Read the model definition and answer for the solid it produces. Units are mm, in the model's axes. Face numbers are marked on the shaded views. A direction names the side the tool comes from. Coordinates: 2 decimals unless noted, no trailing zeros. Order: outer loops, then holes, each group sorted by start corner. A loop starts at its lowest first (then second) coordinate and runs counter-clockwise, first axis right, second up. Notation, with made-up numbers: M 50,4 L 59,4 A19 ccw 59,12 Z; hole C 85,-6.75 d3. An arc over 180 degrees is marked long. Use a Markdown table: item, result. Add a question column.
1) The mould has two halves that part along Z. Classify the marked faces 1, 2 and 3: released by +Z, released by -Z, zero draft, split by the parting line, or undercut.
2) Find the intervals of material crossed by probe 1 along Z at (x, y) = (-53, 19.5); probe 2 along Y at (x, z) = (-15.5, -103.45); probe 3 along X at (y, z) = (31, -102), in increasing order. Write a range as [from, to].
3) Each of these flat-tipped pins is pushed along its axis until it touches: pin 1 Ø2 at (y, z) = (24.5, 22.5) entering from +X; pin 2 Ø10 at (y, z) = (34.5, -17.5) entering from -X; pin 3 Ø1 at (x, z) = (-12, -74.5) entering from +Y. Where does it stop, or does it pass through?
4) For the marked faces 4 and 5, determine the directions among +Z, -Z, +X, -X, +Y, -Y from which every point of the face is accessible in a straight line to the end or side of a thin tool.
5) Find section B-B on y = 39.5. Write down the section's boundary in (x, z).
6) Find section A-A on x = -53. Write down the section's boundary in (y, z), plus the area to 3 significant figures.
7) Find section C-C on z = -27.5. Write down the section's boundary in (x, y), plus the area to 3 significant figures.
Autodesk Inventor part; units mm, degrees
ref_plane "YZ Plane" through (0, 0, 0) normal (1, 0, 0) x (0, 1, 0)
ref_plane "XZ Plane" through (0, 0, 0) normal (0, 1, 0) x (-1, 0, 0)
ref_plane "XY Plane" through (0, 0, 0) normal (0, 0, 1) x (1, 0, 0)
sketch "Boceto1" plane through (0, 0, 0) normal (0, 1, 0) x (-1, 0, 0)
  line L0 (120, 0) -> (60, -103.923)
  line L1 (60, -103.923) -> (-60, -103.923)
  line L2 (-60, -103.923) -> (-120, 0)
  line L3 (-120, 0) -> (-60, 103.923)
  line L4 (-60, 103.923) -> (60, 103.923)
  line L5 (60, 103.923) -> (120, 0)
  point P0 (0, 0)
  point P1 (0, 0)
  dimension "d0" = 120
extrude "Extrusión1" add sketch "Boceto1" along normal blind 3
sketch "Boceto2" plane through (0, 3, 0) normal (0, 1, 0) x (1, 0, 0)
  line L0 (-60, -103.923) -> (60, -103.923)
  line L1 (60, -103.923) -> (120, 0)
  line L2 (120, 0) -> (60, 103.923)
  line L3 (60, 103.923) -> (-60, 103.923)
  line L4 (-60, 103.923) -> (-120, 0)
  line L5 (-120, 0) -> (-60, -103.923)
  line L6 (-58.8453, -101.923) -> (58.8453, -101.923)
  line L7 (58.8453, -101.923) -> (117.6906, 0)
  line L8 (117.6906, 0) -> (58.8453, 101.923)
  line L9 (58.8453, 101.923) -> (-58.8453, 101.923)
  line L10 (-58.8453, 101.923) -> (-117.6906, 0)
  line L11 (-117.6906, 0) -> (-58.8453, -101.923)
  point P0 (0, 0)
  dimension "d3" = 2
extrude "Extrusión2" add sketch "Boceto2" along normal blind 60
sketch "Boceto5" plane through (120, 0, 0) normal (0.866, 0, 0.5) x (0.5, 0, -0.866)
  line L0 (-120, 0) -> (0, 0)
  line L1 (0, 0) -> (0, 63)
  line L2 (-120, 63) -> (0, 63)
  line L3 (-120, 0) -> (-120, 63)
  point P0 (-60, 0)
sketch "Boceto9" plane through (-60, 0, 103.923) normal (-0.866, 0, 0.5) x (0.5, 0, 0.866)
  circle A0 centre (-117, 58.5) radius 1.5
  circle A1 centre (-3, 58.5) radius 1.5
  point P0 (-60, 0)
extrude "Extrusión7" cut sketch "Boceto9" against normal blind 220
sketch "Boceto10" plane through (-120, 0, 0) normal (-0.866, 0, -0.5) x (-0.5, 0, 0.866)
  line L0 (-120, 0) -> (0, 0)
  line L1 (0, 0) -> (0, 63)
  line L2 (-120, 63) -> (0, 63)
  line L3 (-120, 0) -> (-120, 63)
  line L4 (-120, 63) -> (-120, 31.5)
  line L5 (-120, 31.5) -> (-60, 31.5)
  line L6 (-60, 31.5) -> (-60, 0)
  dimension "d19" = 31.5
  dimension "d20" = 60
sketch "Boceto12" plane through (60, 0, -103.923) normal (0, 0, -1) x (-1, 0, 0)
  line L0 (120, 0) -> (120, 63)
  line L1 (120, 31.5) -> (60, 31.5)
  line L2 (60, 31.5) -> (60, 0)
  dimension "d23" = 60
sketch "Boceto13" plane through (60, 0, -103.923) normal (0, 0, -1) x (-1, 0, 0)
  circle A0 centre (44.5, 31.5) radius 1.25
  circle A1 centre (75.5, 31.5) radius 1.25
  point P0 (60, 0)
extrude "Extrusión9" cut sketch "Boceto13" against normal blind 220
sketch "Boceto14" plane through (60, 0, -103.923) normal (0.866, 0, -0.5) x (-0.5, 0, -0.866)
  line L0 (-60, 0) -> (-60, 31.5)
  line L1 (-60, 31.5) -> (0, 31.5)
  dimension "d26" = 31.5
sketch "Boceto15" plane through (60, 0, -103.923) normal (0.866, 0, -0.5) x (-0.5, 0, -0.866)
  circle A0 centre (-75.5, 31.5) radius 1.25
  circle A1 centre (-44.5, 31.5) radius 1.25
  point P0 (-60, 0)
extrude "Extrusión10" cut sketch "Boceto15" against normal blind 220
sketch "Boceto16" plane through (120, 0, 0) normal (0.866, 0, 0.5) x (0.5, 0, -0.866)
  line L0 (-60, 0) -> (-60, 31.5)
  line L1 (-60, 31.5) -> (0, 31.5)
  line L2 (0, 0) -> (0, 63)
  dimension "d29" = 31.5
sketch "Boceto17" plane through (120, 0, 0) normal (0.866, 0, 0.5) x (0.5, 0, -0.866)
  circle A0 centre (-75.5, 31.5) radius 1.25
  circle A1 centre (-44.5, 31.5) radius 1.25
  point P0 (-60, 0)
extrude "Extrusión11" cut sketch "Boceto17" against normal blind 220
properties part number "BaseHEX"
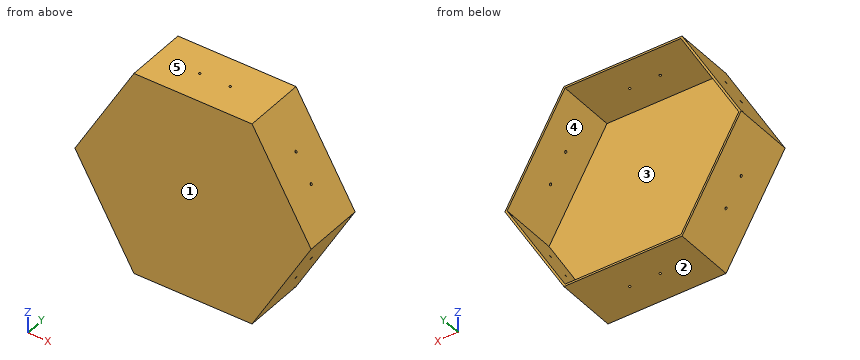
Check result:
| question | item | result |
|---|---|---|
| 1 | face 1 | zero draft |
| 1 | face 2 | released by -Z |
| 1 | face 3 | undercut |
| 2 | probe 1 | z = [-103.92, -101.92], [101.92, 103.92] |
| 2 | probe 2 | y = [0, 30.25], [32.75, 63] |
| 2 | probe 3 | x = [-61.11, -16.65], [-14.35, 14.35], [16.65, 61.11] |
| 3 | pin 1 | stops at x = 107.59 |
| 3 | pin 2 | stops at x = -112.78 |
| 3 | pin 3 | stops at y = 3 |
| 4 | face 4 | +Y |
| 4 | face 5 | +Z, +X, -X, +Y, -Y |
| 5 | outline | M -120,0 L -60,-103.92 L 60,-103.92 L 120,0 L 60,103.92 L -60,103.92 Z; hole M -117.69,0 L -58.85,-101.92 L 58.85,-101.92 L 117.69,0 L 58.85,101.92 L -58.85,101.92 Z |
| 6 | outline | M 0,-103.92 L 63,-103.92 L 63,-101.92 L 3,-101.92 L 3,101.92 L 63,101.92 L 63,103.92 L 0,103.92 Z |
| 6 | area | 864 mm2 |
| 7 | outline | M -104.12,0 L 104.12,0 L 104.12,63 L 101.81,63 L 101.81,3 L -101.81,3 L -101.81,63 L -104.12,63 Z |
| 7 | area | 902 mm2 |
